Autodesk Inventor part; units mm, degrees
ref_plane "YZ Plane" through (0, 0, 0) normal (1, 0, 0) x (0, 1, 0)
ref_plane "XZ Plane" through (0, 0, 0) normal (0, 1, 0) x (-1, 0, 0)
ref_plane "XY Plane" through (0, 0, 0) normal (0, 0, 1) x (1, 0, 0)
sketch "スケッチ1" plane through (0, 0, 0) normal (0, 0, 1) x (1, 0, 0)
  line L0 (-25.9808, -15) -> (25.9808, -15)
  line L1 (25.9808, -15) -> (25.9808, 15)
  line L2 (25.9808, 15) -> (-25.9808, 15)
  line L3 (-25.9808, 15) -> (-25.9808, -15)
  line L4 (-25.9808, -15) -> (25.9808, 15) construction
  line L5 (25.9808, -15) -> (-25.9808, 15) construction
  line L6 (-25.9808, 15) -> (25.9808, 45)
  line L7 (25.9808, 45) -> (25.9808, 15)
  line L8 (-25.9808, 15) -> (-30.9808, 23.6603)
  line L9 (-30.9808, 23.6603) -> (-22.3205, 28.6603)
  line L10 (-22.3205, 28.6603) -> (-17.3205, 20)
  line L11 (8.6603, 35) -> (3.6603, 43.6603)
  line L12 (3.6603, 43.6603) -> (12.3205, 48.6603)
  line L13 (12.3205, 48.6603) -> (17.3205, 40)
  point P0 (0, 0)
  dimension "d0" = 60
  dimension "d1" = 30
  dimension "d2" = 30
  dimension "d3" = 30
  dimension "d4" = 10
  dimension "d5" = 10
  dimension "d6" = 10
  dimension "d7" = 30
extrude "押し出し1" add sketch "スケッチ1" along normal mid plane 5
sketch "スケッチ2" plane through (0, 0, 2.5) normal (0, 0, 1) x (1, 0, 0)
  line L0 (-30.9808, 23.6603) -> (-25.9808, 15)
  line L1 (-25.9808, 15) -> (-25.9808, -15)
  line L2 (-25.9808, -15) -> (25.9808, -15)
  line L3 (25.9808, -15) -> (25.9808, 45)
  line L4 (25.9808, 45) -> (17.3205, 40)
  line L5 (17.3205, 40) -> (12.3205, 48.6603)
  line L6 (12.3205, 48.6603) -> (3.6603, 43.6603)
  line L7 (3.6603, 43.6603) -> (8.6603, 35)
  line L8 (8.6603, 35) -> (-17.3205, 20)
  line L9 (-17.3205, 20) -> (-22.3205, 28.6603)
  line L10 (-22.3205, 28.6603) -> (-30.9808, 23.6603)
  point P0 (0, 0)
  point P1 (-24.1506, 21.8301)
  point P2 (10.4904, 41.8301)
  dimension "d10" = 5
  dimension "d11" = 5
  dimension "d12" = 5
  dimension "d13" = 5
hole "穴1" at (-24.1506, 21.8301, 2.5) at (10.4904, 41.8301, 2.5) direction (0, 0, -1) diameter 4.3 end through all
sketch "スケッチ4" plane through (0, 0, 2.5) normal (0, 0, 1) x (1, 0, 0)
  line L0 (-25.9808, -15) -> (25.9808, -15)
  line L1 (25.9808, -15) -> (25.9808, 45)
  point P0 (0, 0)
  point P1 (10.9808, 15)
  dimension "d30" = 30
  dimension "d31" = 15
hole "穴2" at (10.9808, 15, 2.5) direction (0, 0, -1) diameter 3.1 end through all
sketch "スケッチ5" plane through (0, 0, 2.5) normal (0, 0, 1) x (1, 0, 0)
  line L0 (-25.9808, 15) -> (-25.9808, -15)
  line L1 (-25.9808, -15) -> (25.9808, -15)
  line L2 (25.9808, -15) -> (25.9808, 45)
  point P0 (0, 0)
  point P1 (-20.9808, 10)
  point P2 (-20.9808, -10)
  point P3 (20.9808, -10)
  dimension "d39" = 5
  dimension "d40" = 5
  dimension "d41" = 5
  dimension "d42" = 20
  dimension "d43" = 5
  dimension "d44" = 5
hole "穴3" at (-20.9808, 10, 2.5) at (-20.9808, -10, 2.5) at (20.9808, -10, 2.5) direction (0, 0, -1) diameter 3.3 end through all
sketch "スケッチ7" plane through (0, 0, -2.5) normal (0, 0, -1) x (-1, 0, 0)
  line L0 (-25.9808, -15) -> (25.9808, -15)
  line L1 (-25.9808, 45) -> (-25.9808, -15)
  line L2 (-5.9808, -10) -> (4.0192, -10)
  line L3 (4.0192, -10) -> (4.0192, -12)
  line L4 (4.0192, -12) -> (-5.9808, -12)
  line L5 (-5.9808, -12) -> (-5.9808, -10)
  line L6 (-5.9808, -10) -> (4.0192, -10)
  line L7 (4.0192, -10) -> (4.0192, -8)
  line L8 (4.0192, -8) -> (-5.9808, -8)
  line L9 (-5.9808, -8) -> (-5.9808, -10)
  point P0 (0, 0)
  dimension "d52" = 5
  dimension "d53" = 20
  dimension "d54" = 5
  dimension "d55" = 10
  dimension "d56" = 2
  dimension "d57" = 2
extrude "押し出し3" cut sketch "スケッチ7" against normal blind 10
fillet "フィレット1" radius 2 2 edges at (5.9808, -10, 2.5) (5.9808, -10, -2.5)
fillet "フィレット2" radius 2 7 edges at (17.3205, 40, 0) (25.9808, 45, 0) (-17.3205, 20, 0) (8.6603, 35, 0) (-25.9808, 15, 0) (25.9808, -15, 0) (-25.9808, -15, 0)
sketch "スケッチ8" plane through (0, 0, -2.5) normal (0, 0, -1) x (-1, 0, 0)
  arc A0 (23.9808, -15) -> (25.9808, -13) centre (23.9808, -13) ccw
  line L0 (25.9808, -13) -> (25.9808, 14.4641)
  arc A1 (26.2487, 15.4641) -> (25.9808, 14.4641) centre (27.9808, 14.4641) ccw
  line L1 (26.2487, 15.4641) -> (30.9808, 23.6603)
  line L2 (30.9808, 23.6603) -> (22.3205, 28.6603)
  line L3 (22.3205, 28.6603) -> (18.3205, 21.7321)
  arc A2 (15.5885, 21) -> (18.3205, 21.7321) centre (16.5885, 22.7321) ccw
  line L4 (15.5885, 21) -> (-6.9282, 34)
  arc A3 (-7.6603, 36.7321) -> (-6.9282, 34) centre (-5.9282, 35.7321) ccw
  line L5 (-7.6603, 36.7321) -> (-3.6603, 43.6603)
  line L6 (-3.6603, 43.6603) -> (-12.3205, 48.6603)
  line L7 (-12.3205, 48.6603) -> (-16.3205, 41.7321)
  arc A4 (-19.0526, 41) -> (-16.3205, 41.7321) centre (-18.0526, 42.7321) ccw
  line L8 (-19.0526, 41) -> (-22.9808, 43.2679)
  arc A5 (-22.9808, 43.2679) -> (-25.9808, 41.5359) centre (-23.9808, 41.5359) ccw
  line L9 (-25.9808, 41.5359) -> (-25.9808, -13)
  arc A6 (-25.9808, -13) -> (-23.9808, -15) centre (-23.9808, -13) ccw
  line L10 (-23.9808, -15) -> (23.9808, -15)
  circle A7 centre (24.1506, 21.8301) radius 2.15
  circle A8 centre (-10.4904, 41.8301) radius 2.15
  circle A9 centre (-10.9808, 15) radius 1.55
  circle A10 centre (20.9808, 10) radius 1.65
  circle A11 centre (20.9808, -10) radius 1.65
  circle A12 centre (-20.9808, -10) radius 1.65
  line L11 (-7.9808, -8) -> (4.0192, -8)
  line L12 (4.0192, -8) -> (4.0192, -12)
  line L13 (4.0192, -12) -> (-7.9808, -12)
  line L14 (-7.9808, -8) -> (-7.9808, -12)
  circle A13 centre (-10.4904, 41.8301) radius 5
  circle A14 centre (24.1506, 21.8301) radius 5
  point P0 (0, 0)
  point P1 (19.8205, 24.3301)
  point P2 (26.6506, 26.1603)
  point P3 (28.4808, 19.3301)
  point P4 (-14.8205, 44.3301)
  point P5 (-7.9904, 46.1603)
  point P6 (-6.1603, 39.3301)
extrude "押し出し4" cut sketch "スケッチ8" against normal blind 10 contours A14 L2 L1 | L3 L2 A14 | L7 L6 A13 | L6 L5 A13
equation "\"d5\" = d4"
equation "\"d6\" = d4"
equation "\"d54\" = d52"
equation "\"d56\" = d57"
properties part number "ベースパーツ1"
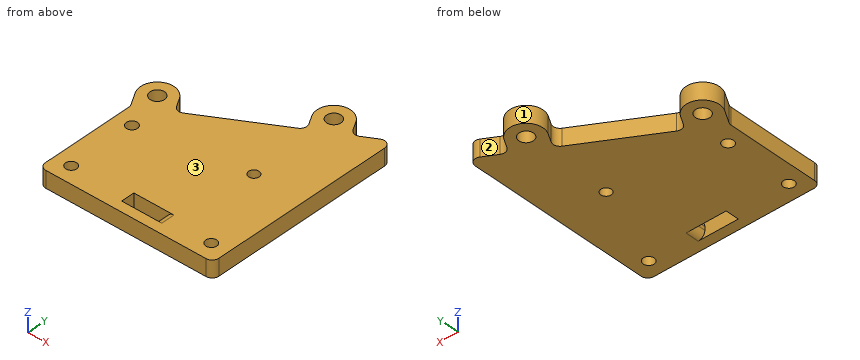
The listing builds one solid part. Answer for the finished solid, in the listing's coordinates (mm). Face numbers are marked on the shaded views. Coordinates: 2 decimals unless noted, no trailing zeros. Write each loop counter-clockwise with the first axis right and the second up, starting at its lowest first coordinate (ties: lowest second). Pieces come first, ordered by that corner, then holes. Notation, with made-up numbers: M 3,-9.5 L 38,-9.5 A30 cw 38,24.5 Z; hole C -2.75,-1 d10. An arc over 180 degrees is marked long. Use a Markdown table: item, result. Add a question column.
1. Section D-D (z = -1.25) is taken. Give the vertices of the cut face in (x, y), plus the area to 3 significant figures.
2. Straight lines are drawn through the part: line 1 along X through (y, z) = (-10, 1.45); line 2 along Y through (x, z) = (-24, -0.4); line 3 along X through (y, z) = (-10, -1.25). For each, find the intervals that lie inside material, in ascending order. Write a range as [from, to].
3. Section B-B (y = -10) is taken. Give the vertices of the cut face in (x, z), plus the area to 3 significant figures.
4. For a pull along X with two mould halves and no side action, classify the marked faces 1, 2 and 3 as +X half, -X half, draft (parallel to the pull), parting line (faces both ways), or undercut.
5. Given P1, Ø5.5, axis at x = -24.15, y = 21.83, coming from the +Z side; P2, Ø1, axis at y = 19, z = -0.5, coming from the -X side; P3, Ø3.5, axis at x = 10.49, y = 41.83, coming from the +Z side; P4, Ø1.5, axis at y = -4.5, z = 1, coming from the -X side, each flat-ended and moving along its own axis, determine where each tip first touches the part or whether it passes through.
6. Section A-A (y = 10) is taken. Give the vertices of the cut face in (x, z).
7. Section C-C (x = 3) is taken. Give the vertices of the cut face in (y, z).
Data:
| question | item | result |
|---|---|---|
| 1 | outline | M -28.48,19.33 L -26.25,15.46 A2 cw -25.98,14.46 L -25.98,-13 A2 ccw -23.98,-15 L 23.98,-15 A2 ccw 25.98,-13 L 25.98,41.54 A2 ccw 22.98,43.27 L 19.05,41 A2 cw 16.32,41.73 L 14.82,44.33 A5 ccw 6.16,39.33 L 7.66,36.73 A2 cw 6.93,34 L -15.59,21 A2 cw -18.32,21.73 L -19.82,24.33 A5 ccw Z; hole C -24.15,21.83 d4.3; hole C -20.98,-10 d3.3; hole C -20.98,10 d3.3; hole M -4.02,-12 L 6.13,-12 L 6.13,-8 L -4.02,-8 Z; hole C 10.49,41.83 d4.3; hole C 10.98,15 d3.1; hole C 20.98,-10 d3.3 |
| 1 | area | 2,410 mm2 |
| 2 | line 1 | x = [-25.98, -22.63], [-19.33, -4.02], [6.22, 19.33], [22.63, 25.98] |
| 2 | line 2 | y = [-15, 19.69], [23.97, 26.83] |
| 2 | line 3 | x = [-25.98, -22.63], [-19.33, -4.02], [6.13, 19.33], [22.63, 25.98] |
| 3 | outline | M -25.98,-2.5 L -22.63,-2.5 L -22.63,2.5 L -25.98,2.5 Z; M -19.33,-2.5 L -4.02,-2.5 L -4.02,2.5 L -19.33,2.5 Z; M 5.98,-0.5 A2 ccw 7.98,-2.5 L 19.33,-2.5 L 19.33,2.5 L 7.98,2.5 A2 ccw 5.98,0.5 Z; M 22.63,-2.5 L 25.98,-2.5 L 25.98,2.5 L 22.63,2.5 Z |
| 3 | area | 175 mm2 |
| 4 | face 1 | parting line |
| 4 | face 2 | undercut |
| 4 | face 3 | draft |
| 5 | P1 | stops at z = 2.5 |
| 5 | P2 | stops at x = -28.57 |
| 5 | P3 | passes through |
| 5 | P4 | stops at x = -25.98 |
| 6 | outline | M -25.98,-2.5 L -22.63,-2.5 L -22.63,2.5 L -25.98,2.5 Z; M -19.33,-2.5 L 25.98,-2.5 L 25.98,2.5 L -19.33,2.5 Z |
| 7 | outline | M -15,-2.5 L -12,-2.5 L -12,2.5 L -15,2.5 Z; M -8,-2.5 L 31.73,-2.5 L 31.73,2.5 L -8,2.5 Z |
